Could you check a few things on this model? Use its own coordinates, in mm. Face numbers are marked on the shaded views. A direction names the side the tool comes from. Coordinates: 2 decimals unless noted, no trailing zeros. Loops run counter-clockwise (first coordinate to the right, second up) from the corner with the lowest first, then second, coordinate; pieces in that order, holes last.
1) Thinking about a two-plate mould opening in X: for the marked faces 1, 2, 3 and 4, which applies, released by +X, released by -X, zero draft, split by the parting line, or undercut?
2) Imagine slicing it at D-D on z = 5.75. Please give me the cut outline in (x, y).
3) Will these pins go through, and if not, where does the flat tip stop? P1, Ø3, axis at x = 15.5, z = -6, coming from the +Y side; P2, Ø1.6, axis at x = -2, y = 1, coming from the +Z side; P3, Ø2, axis at x = -8.5, z = -10, coming from the -Y side; P4, Ø1, axis at x = 21, z = 1.5, coming from the +Y side.
4) Imagine slicing it at C-C on y = 15.5. Please give me the cut outline in (x, z).
5) Imagine slicing it at B-B on z = -9.75. Please give me the cut outline in (x, y), plus the area to 3 significant figures.
6) If I drill on line 1 along X through (y, z) = (11.75, 11.25); line 2 along X through (y, z) = (20, -5); line 3 along Y through (x, z) = (-10.5, -5), over which ranges is the centre line in solid material (lowest first)?
7) For the marked faces 5 and 6, which set-ups out of +Z, -Z, +X, -X, +Y, -Y let a thin tool reach every point of the face, with its end or its side?
8) Imagine slicing it at A-A on y = 10.5. Please give me the cut outline in (x, z).
```python
from build123d import *

# Parameters (mm, degrees)
SKETCH2_W           = 44
SKETCH2_H           = 29
BOSS_EXTRUDE1_DEPTH = 23
SKETCH3_W           = 40
SKETCH3_H           = 25
CUT_EXTRUDE1_DEPTH  = 21
SKETCH4_W           = 20.7
SKETCH4_H           = 2
CUT_EXTRUDE2_DEPTH  = 33
SKETCH5_W           = 30
SKETCH5_H           = 12.3
CUT_EXTRUDE3_DEPTH  = 2
CUT_EXTRUDE5_DEPTH  = 2
SKETCH11_W          = 3.9
SKETCH11_H          = 8.6
SKETCH11_W_2        = 7
SKETCH11_H_2        = 1.5
CUT_EXTRUDE6_DEPTH  = 2
SKETCH13_W          = 8
SKETCH13_H          = 6
CUT_EXTRUDE8_DEPTH  = 2
SKETCH14_W          = 44
SKETCH14_H          = 2
CUT_EXTRUDE9_DEPTH  = 23


with BuildPart() as part:
    # Sketch2 → Boss-Extrude1 (new body)
    with BuildSketch(Plane(origin=(0, 0, 0), x_dir=(1, 0, 0), z_dir=(0, 1, 0))):
        Rectangle(SKETCH2_W, SKETCH2_H)
    extrude(amount=BOSS_EXTRUDE1_DEPTH)

    # Sketch3 → Cut-Extrude1 (cut)
    with BuildSketch(Plane(origin=(0, 23, 0), x_dir=(1, 0, 0), z_dir=(0, 1, 0))):
        Rectangle(SKETCH3_W, SKETCH3_H)
    extrude(amount=-CUT_EXTRUDE1_DEPTH, mode=Mode.SUBTRACT)

    # Sketch4 → Cut-Extrude2 (cut)
    with BuildSketch(Plane.XY.offset(14.5)):
        with Locations((0.25, 18.2)):
            Rectangle(SKETCH4_W, SKETCH4_H)
    extrude(amount=-CUT_EXTRUDE2_DEPTH, mode=Mode.SUBTRACT)

    # Sketch5 → Cut-Extrude3 (cut)
    with BuildSketch(Plane.XY.offset(14.5)):
        with Locations((0, 8.15)):
            Rectangle(SKETCH5_W, SKETCH5_H)
    extrude(amount=-CUT_EXTRUDE3_DEPTH, mode=Mode.SUBTRACT)

    # Sketch8 → Cut-Extrude5 (cut)
    with BuildSketch(Plane(origin=(22, 0, 0), x_dir=(0, 0, -1), z_dir=(1, 0, 0))):
        Polygon((-12.5, 17), (-4, 17), (-4, 13.5), (4, 13.5), (4, 17), (12.5, 17), (12.5, 23), (-12.5, 23), align=None)
    extrude(amount=-CUT_EXTRUDE5_DEPTH, mode=Mode.SUBTRACT)

    # Sketch11 → Cut-Extrude6 (cut)
    with BuildSketch(Plane(origin=(0, 0, -14.5), x_dir=(-1, 0, 0), z_dir=(0, 0, -1))):
        with Locations((-18.05, 6.3)):
            Rectangle(SKETCH11_W, SKETCH11_H)
        with Locations((12.4, 2.75)):
            Rectangle(SKETCH11_W_2, SKETCH11_H_2)
    extrude(amount=-CUT_EXTRUDE6_DEPTH, mode=Mode.SUBTRACT)

    # Sketch13 → Cut-Extrude8 (cut)
    with BuildSketch(Plane(origin=(0, 2, 0), x_dir=(1, 0, 0), z_dir=(0, 1, 0))):
        with Locations((-11, -9.5)):
            Rectangle(SKETCH13_W, SKETCH13_H)
        with Locations((0, -9.5)):
            Rectangle(SKETCH13_W, SKETCH13_H)
        with Locations((11, 9.5)):
            Rectangle(SKETCH13_W, SKETCH13_H)
        with Locations((11, -9.5)):
            Rectangle(SKETCH13_W, SKETCH13_H)
        with Locations((-11, 9.5)):
            Rectangle(SKETCH13_W, SKETCH13_H)
        with Locations((0, 9.5)):
            Rectangle(SKETCH13_W, SKETCH13_H)
    extrude(amount=-CUT_EXTRUDE8_DEPTH, mode=Mode.SUBTRACT)

    # Sketch14 → Cut-Extrude9 (cut)
    with BuildSketch(Plane(origin=(0, 23, 0), x_dir=(1, 0, 0), z_dir=(0, 1, 0))):
        with Locations((0, -13.5)):
            Rectangle(SKETCH14_W, SKETCH14_H)
        with Locations((0, 13.5)):
            Rectangle(SKETCH14_W, SKETCH14_H)
    extrude(amount=-CUT_EXTRUDE9_DEPTH, mode=Mode.SUBTRACT)


solid = part.part
```
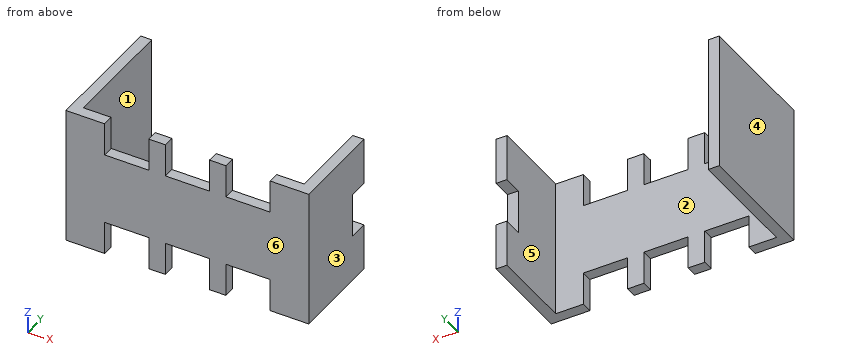
Filled in:
1. face 1: undercut
1. face 2: undercut
1. face 3: released by +X
1. face 4: released by -X
2. outline: (-22, 0) - (22, 0) - (22, 17) - (20, 17) - (20, 2) - (-20, 2) - (-20, 23) - (-22, 23) - close
3. P1: stops at y = 2
3. P2: stops at z = 6.5
3. P3: passes through
3. P4: stops at y = 13.5
4. outline: (-22, -12.5) - (-20, -12.5) - (-20, 12.5) - (-22, 12.5) - close; (20, -12.5) - (22, -12.5) - (22, -4) - (20, -4) - close; (20, 4) - (22, 4) - (22, 12.5) - (20, 12.5) - close
5. outline: (-22, 0) - (-15, 0) - (-15, 2) - (-20, 2) - (-20, 23) - (-22, 23) - close; (-7, 0) - (-4, 0) - (-4, 2) - (-7, 2) - close; (4, 0) - (7, 0) - (7, 2) - (4, 2) - close; (15, 0) - (22, 0) - (22, 17) - (20, 17) - (20, 2) - (15, 2) - close
5. area: 112 mm2
6. line 1: x = -22 to -20, 20 to 22
6. line 2: x = -22 to -20
6. line 3: y = 0 to 2
7. face 5: +Z, -Z, +Y
7. face 6: +Z, -Z, +X, -X, -Y
8. outline: (-22, -12.5) - (-20, -12.5) - (-20, 12.5) - (-22, 12.5) - close; (20, -12.5) - (22, -12.5) - (22, 12.5) - (20, 12.5) - close
